Could you check a few things on this model? Use its own coordinates, in mm. Face numbers are marked on the shaded views. Round coordinates to 2 decimals unless told otherwise and drop trailing zeros. Write each loop counter-clockwise with the first axis right and the second up, starting at its lowest first coordinate (ties: lowest second). Pieces come first, ordered by that corner, then holes.
```python
from build123d import *

# Parameters (mm, degrees)
F1_DEPTH = 9.525


with BuildPart() as f1:
    # F0 (on Front) → F1 (new body)
    with BuildSketch(Plane.XZ):
        with BuildLine():
            Line((13.503937, 61.43969), (-41.496063, 61.43969))
            ThreePointArc((-41.496063, 61.43969), (-48.567131, 58.510758), (-51.496063, 51.43969))
            Line((-51.496063, 51.43969), (-51.496063, -28.56031))
            ThreePointArc((-51.496063, -28.56031), (-48.567131, -35.631378), (-41.496063, -38.56031))
            Line((-41.496063, -38.56031), (13.503937, -38.56031))
            ThreePointArc((13.503937, -38.56031), (20.575005, -35.631378), (23.503937, -28.56031))
            Line((23.503937, -28.56031), (23.503937, 51.43969))
            ThreePointArc((23.503937, 51.43969), (20.575005, 58.510758), (13.503937, 61.43969))
        make_face()
        Polygon((-23.996063, -9.495226), (-3.996063, -9.495226), (-3.996063, -19.020226), (-13.996063, -19.020226), (-23.996063, -19.020226), align=None, mode=Mode.SUBTRACT)
        Polygon((-23.996063, 41.899607), (-13.996063, 41.899607), (-3.996063, 41.899607), (-3.996063, 32.374607), (-23.996063, 32.374607), align=None, mode=Mode.SUBTRACT)
    extrude(amount=F1_DEPTH)


solid = f1.part
```
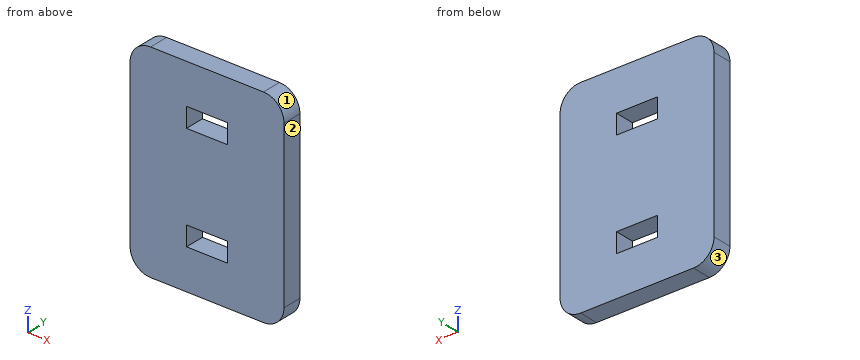
Q1. If I drill on L1, parallel to Z at x = -18, y = -0.75; L2, parallel to X at y = -1.75, z = 37.5; L3, parallel to X at y = -5, z = -32, over which ranges is the centre line in solid material (lowest first)?
Q2. Imagine slicing it at C-C, the plane z = -14.5. Write out the boundary of the cut face in (x, y) (3 decimals).
Q3. Imagine slicing it at A-A, the plane x = -16. Write out the boundary of the cut face in (y, z) (3 decimals), then the cut area to 3 significant figures.
Q4. We'd pull the mould along Z, two halves only. Please class the marked faces 1, 2 and 3: pulls with the +Z half, pulls with the -Z half, needs draft (parallel to the pull), parting line crosses it, or undercut.
Q5. Imagine slicing it at B-B, the plane y = -5. Write out the boundary of the cut face in (x, z).
Results found:
1. L1: z = -38.56 to -19.02, -9.5 to 32.37, 41.9 to 61.44
1. L2: x = -51.5 to -24, -4 to 23.5
1. L3: x = -50.89 to 22.89
2. outline: (-51.496, -9.525) - (-23.996, -9.525) - (-23.996, 0) - (-51.496, 0) - close; (-3.996, -9.525) - (23.504, -9.525) - (23.504, 0) - (-3.996, 0) - close
3. outline: (-9.525, -38.56) - (0, -38.56) - (0, -19.02) - (-9.525, -19.02) - close; (-9.525, -9.495) - (0, -9.495) - (0, 32.375) - (-9.525, 32.375) - close; (-9.525, 41.9) - (0, 41.9) - (0, 61.44) - (-9.525, 61.44) - close
3. area: 771 mm2
4. face 1: pulls with the +Z half
4. face 2: needs draft
4. face 3: pulls with the -Z half
5. outline: (-51.5, -28.56) arc R10 ccw to (-41.5, -38.56) - (13.5, -38.56) arc R10 ccw to (23.5, -28.56) - (23.5, 51.44) arc R10 ccw to (13.5, 61.44) - (-41.5, 61.44) arc R10 ccw to (-51.5, 51.44) - close; hole (-24, -19.02) - (-4, -19.02) - (-4, -9.5) - (-24, -9.5) - close; hole (-24, 32.37) - (-4, 32.37) - (-4, 41.9) - (-24, 41.9) - close
